Input: part model. Units: mm. Frame: model coordinates. A direction names the side the tool comes from. Coordinates: 2 decimals unless noted, no trailing zeros. Loops run counter-clockwise (first coordinate to the right, second up) from the corner with the lowest first, then second, coordinate; pieces in that order, holes last.
Autodesk Inventor part; units mm, degrees
ref_plane "YZ Plane" through (0, 0, 0) normal (1, 0, 0) x (0, 1, 0)
ref_plane "XZ Plane" through (0, 0, 0) normal (0, 1, 0) x (-1, 0, 0)
ref_plane "XY Plane" through (0, 0, 0) normal (0, 0, 1) x (1, 0, 0)
sketch "스케치1" plane through (0, 0, 0) normal (0, 1, 0) x (-1, 0, 0)
  line L0 (0, 0) -> (-25, 0)
  line L1 (-25, 0) -> (-25, -24)
  line L2 (-25, -24) -> (0, -24)
  line L3 (0, -24) -> (0, 0)
  circle A0 centre (-2, -22) radius 1
  circle A1 centre (-23, -22) radius 1
  circle A2 centre (-23, -9.5) radius 1
  circle A3 centre (-2, -9.5) radius 1
  line L4 (-8.5, -13.5) -> (-16.5, -13.5)
  line L5 (-16.5, -13.5) -> (-16.5, -5.5)
  line L6 (-16.5, -5.5) -> (-8.5, -5.5)
  line L7 (-8.5, -5.5) -> (-8.5, -13.5)
  circle A4 centre (-12.5, -9.5) radius 4
  line L8 (-2.1, 0) -> (-22.9, 0)
  line L9 (-22.9, 0) -> (-22.9, -5.5)
  line L10 (-22.9, -5.5) -> (-2.1, -5.5)
  line L11 (-2.1, -5.5) -> (-2.1, 0)
  point P0 (-12.5, 0)
  point P1 (-16.5, -9.5)
  point P2 (-12.5, -5.5)
  point P3 (-8.5, -9.5)
  point P4 (-12.5, -13.5)
  dimension "d0" = 25
  dimension "d1" = 24
  dimension "d2" = 2
  dimension "d3" = 2
  dimension "d4" = 2
  dimension "d5" = 2
  dimension "d6" = 2
  dimension "d8" = 2
  dimension "d9" = 2
  dimension "d10" = 2
  dimension "d12" = 2
  dimension "d15" = 12.5
  dimension "d16" = 9.5
  dimension "d17" = 2
  dimension "d18" = 12.5
  dimension "d19" = 9.5
  dimension "d20" = 8
  dimension "d21" = 8
  dimension "d22" = 8.5
  dimension "d23" = 8.5
  dimension "d24" = 5.5
  dimension "d25" = 21
  dimension "d26" = 8
  dimension "d27" = 20.8
  dimension "d28" = 5.5
extrude "돌출1" add sketch "스케치1" along normal blind 0.95 contours L3 L2 L1 L0 L9 L10 L5 L4 L7 L11 | L11 L10 L6 L9 L0
extrude "돌출2" add sketch "스케치1" along normal blind 3.95 contours L7 A4 L6 | L6 A4 L5 | L7 L4 A4 | A4 L4 L5
extrude "돌출3" add sketch "스케치1" along normal blind 5.2 contours A4
extrude "돌출4" add sketch "스케치1" against normal blind 2.8 contours L11 L10 L6 L9 L0
sketch "스케치2" plane through (0, 0.95, 0) normal (0, 0, 1) x (1, 0, 0)
  line L0 (4.4, -2.22) -> (20.6, -2.22)
  line L1 (20.6, -2.22) -> (20.6, -2.72)
  line L2 (20.6, -2.72) -> (4.4, -2.72)
  line L3 (4.4, -2.72) -> (4.4, -2.22)
  line L4 (0, -0.95) -> (2.1, -0.95)
  line L5 (2.1, -0.95) -> (2.1, -3.75)
  line L6 (22.9, -0.95) -> (22.9, -3.75)
  point P0 (4.4, -2.47)
  point P1 (20.6, -2.47)
  dimension "d37" = 16.2
  dimension "d38" = 0.5
  dimension "d39" = 1.27
  dimension "d40" = 2.3
  dimension "d41" = 2.3
  dimension "d42" = 2.1
extrude "돌출5" cut sketch "스케치2" against normal blind 3
properties part number "r_camera v2"
Item 1: Section query B-B (y = -0.5). Output: boundary loops of the cut face in (x, z).
Result:
outline: (2.1, -5.5) - (22.9, -5.5) - (22.9, 0) - (2.1, 0) - close
Item 2: Section query D-D (y = 2.25). Output: boundary loops of the cut face in (x, z).
Result:
outline: (8.5, -13.5) - (16.5, -13.5) - (16.5, -5.5) - (8.5, -5.5) - close
Item 3: Reachability of faces 1 (the face through (13, 2, -5.5)), 2 (the face through (22.9, -1, -3)), 3 (the face through (9, 3.95, -6)), 4 (the face through (16, 3.95, -13)) from +Z, -Z, +X, -X, +Y, -Y: full face, straight path, thin tool, end or side. Return the list, or none.
Result:
face 1: +Z, +X, -X, +Y
face 2: +Z, -Z, +X, -Y
face 3: +Z, -X, +Y
face 4: -Z, +X, +Y
Item 4: Section query A-A (x = 18.25). Output: boundary loops of the cut face in (y, z).
Result:
outline: (-2.8, -5.5) - (0, -5.5) - (0, -24) - (0.95, -24) - (0.95, 0) - (-1.27, 0) - (-1.27, -3) - (-1.77, -3) - (-1.77, 0) - (-2.8, 0) - close
Item 5: Contact query for flat-ended pins moving along their axis: P1, Ø3, axis at x = 2, z = -22, coming from the -Y side; P2, Ø2, axis at x = 16.5, y = 1, coming from the +Z side; P3, Ø2, axis at x = 5.5, y = 3.5, coming from the +Z side; P4, Ø0.6, axis at y = -1.5, z = -1, coming from the -X side. Output: stop coordinate, or through.
Result:
P1: stops at y = 0
P2: stops at z = 0
P3: passes through
P4: stops at x = 2.1
Item 6: Line query: L1, parallel to Z at x = 2, y = 0.6; L2, parallel to Y at x = 19.75, z = -1; L3, parallel to Y at x = 7.75, z = -11.75. Output: solid intervals per line, ascending.
Result:
L1: z = -24 to -23, -21 to -10.5, -8.5 to 0
L2: y = -2.8 to -1.77, -1.27 to 0.95
L3: y = 0 to 0.95
Item 7: Section query C-C (x = 15). Output: boundary loops of the cut face in (y, z), then the cut area to 3 significant figures.
Result:
outline: (-2.8, -5.5) - (0, -5.5) - (0, -24) - (0.95, -24) - (0.95, -13.5) - (3.95, -13.5) - (3.95, -12.62) - (5.2, -12.62) - (5.2, -6.38) - (3.95, -6.38) - (3.95, -5.5) - (0.95, -5.5) - (0.95, 0) - (-1.27, 0) - (-1.27, -3) - (-1.77, -3) - (-1.77, 0) - (-2.8, 0) - close
area: 68.5 mm2
Item 8: Mould query, pull axis X, two halves, no side actions, for faces 5 (the face through (23.13, 0.47, -10.49)), 6 (the face through (8.5, 2, -9)), 7 (the face through (9, 3.95, -13)). Classes: +X half, -X half, draft (parallel to the pull), parting line (faces both ways), or undercut.
Result:
face 5: undercut
face 6: -X half
face 7: draft
